Build history of the part. All positions in model axes, mm. A direction names the side the tool comes from. Coordinates: 2 decimals unless noted, no trailing zeros. Loops run counter-clockwise (first coordinate to the right, second up) from the corner with the lowest first, then second, coordinate; pieces in that order, holes last. Notation, with made-up numbers: (86, 56) - (133, 56) arc R18 ccw to (133, 90) - close; hole circle Ø4 at (15, 14). An arc over 180 degrees is marked (long way). One line per item, written item: value.
```python
from build123d import *

# Parameters (mm, degrees)
SKETCH2_R           = 10
BOSS_EXTRUDE1_DEPTH = 8
SKETCH3_R           = 12.5
SKETCH3_R_2         = 7.5
BOSS_EXTRUDE2_DEPTH = 50
BOSS_EXTRUDE3_START = 10
SKETCH4_R           = 12.5
SKETCH4_R_2         = 7.5
BOSS_EXTRUDE3_DEPTH = 10
BOSS_EXTRUDE4_DEPTH = 40
CUT_EXTRUDE1_DEPTH  = 72.52071964
FILLET1_R           = 3


with BuildPart() as part:
    # Sketch2 → Boss-Extrude1 (new body)
    with BuildSketch(Plane(origin=(0, 0, 0), x_dir=(1, 0, 0), z_dir=(0, 1, 0))):
        with BuildLine():
            Line((0, 27.802301255), (0, -12.197698745))
            Line((0, -12.197698745), (19.5, -12.197698745))
            ThreePointArc((19.5, -12.197698745), (39.5, 7.802301255), (19.5, 27.802301255))
            Line((19.5, 27.802301255), (0, 27.802301255))
        make_face()
        with Locations(Location((19.5, 7.802301255, 0), (0, 0, 270))):
            Circle(SKETCH2_R, mode=Mode.SUBTRACT)
    extrude(amount=-BOSS_EXTRUDE1_DEPTH)

    # Sketch3 → Boss-Extrude2 (add)
    with BuildSketch(Plane.XY.offset(12.197698745)):
        with Locations((-8.910855114, -4)):
            Circle(SKETCH3_R)
        with Locations((-8.910855114, -4)):
            Circle(SKETCH3_R_2, mode=Mode.SUBTRACT)
    extrude(amount=-BOSS_EXTRUDE2_DEPTH)

    # Sketch4 → Boss-Extrude3 (add)
    with BuildSketch(Plane.XY.offset(12.197698745).offset(BOSS_EXTRUDE3_START)):
        with Locations((-8.910855114, -4)):
            Circle(SKETCH4_R)
        with Locations((-8.910855114, -4)):
            Circle(SKETCH4_R_2, mode=Mode.SUBTRACT)
    extrude(amount=-BOSS_EXTRUDE3_DEPTH)

    # Sketch6 → Boss-Extrude4 (add)
    with BuildSketch(Plane.XY.offset(12.197698745)):
        Polygon((-18.032516938, -3.352408244), (-55.511163409, 18.285898385), (-51.511163409, 25.214101615), (-14.032516938, 3.575794986), align=None)
    extrude(amount=-BOSS_EXTRUDE4_DEPTH)

    # Sketch7 → Cut-Extrude1 (cut, through all)
    with BuildSketch(Plane(origin=(-1.959764586, -3.394411834, 0), x_dir=(0.866025403784438, -0.500000000000001, 0), z_dir=(0.500000000000001, 0.866025403784438, 0))):
        with BuildLine():
            Line((-47.217026898, 12.802301255), (-27.217026898, 12.802301255))
            ThreePointArc((-27.217026898, 12.802301255), (-22.217026898, 7.802301255), (-27.217026898, 2.802301255))
            Line((-27.217026898, 2.802301255), (-47.217026898, 2.802301255))
            ThreePointArc((-47.217026898, 2.802301255), (-52.217026898, 7.802301255), (-47.217026898, 12.802301255))
        make_face()
    extrude(amount=-CUT_EXTRUDE1_DEPTH, mode=Mode.SUBTRACT)

    # Fillet1
    fillet1_edges = [part.edges().sort_by_distance(p)[0] for p in [
        (-53.511163409, 21.75, -27.802301255),
        (-53.511163409, 21.75, 12.197698745),
    ]]
    fillet(fillet1_edges, radius=FILLET1_R)


solid = part.part
```
Item 1: Pull direction Z, two halves, no side cores. Call faces 1 (the face through (29.415, -3.944, -9.104)), 2 (the face through (25, -8, 1)), 3 (the face through (-52.7, 21.35, 11.34)), 4 (the face through (-49.15, 19.3, -7.69)): released by +Z, released by -Z, zero draft, split by the parting line, or undercut.
Check result:
face 1: undercut
face 2: zero draft
face 3: released by +Z
face 4: undercut
Item 2: Cut at D-D, the plane y = -9. Write the cut outline in (x, z), then the cut area to 3 significant figures.
Check result:
outline: (-20.37, -37.8) - (-14.5, -37.8) - (-14.5, 22.2) - (-20.37, 22.2) - close; (-3.32, -37.8) - (2.55, -37.8) - (2.55, 22.2) - (-3.32, 22.2) - close
area: 704 mm^2
Item 3: Cut at B-B, the plane x = -4. Write the cut outline in (y, z), then the cut area to 3 significant figures.
Check result:
outline: (-15.49, -37.8) - (-9.67, -37.8) - (-9.67, 22.2) - (-15.49, 22.2) - close; (1.67, -37.8) - (7.49, -37.8) - (7.49, 22.2) - (1.67, 22.2) - close
area: 699 mm^2
Item 4: Probe probe 1 along Z at (x, y) = (19, -2); probe 2 along Y at (x, z) = (15, -21); probe 3 along X at (y, z) = (-9.5, -33.5). List the from-to ranges inside material, lowest first. Write a range as from..to.
Check result:
probe 1: z = -27.8..-17.79, 2.19..12.2
probe 2: y = -8..0
probe 3: x = -20.14..-14.01, -3.81..2.31
Item 5: Drop flat-ended pins along their axis: P1, Ø8, axis at y = -3, z = 7, coming from the +X side; P2, Ø18.5, axis at x = -32.5, y = 9, coming from the +Z side; P3, Ø6, axis at x = 20.5, y = 2, coming from the -Z side. Give the stop position or say it passes through.
Check result:
P1: stops at x = 36.33
P2: stops at z = 12.2
P3: stops at z = -27.8
Item 6: Tool access for faces 5 (the face through (-9, -12, 22.198)), 6 (the face through (-34.58, 15.44, -16.41)): list every direction of +Z, -Z, +X, -X, +Y, -Y with a clear straight run to the whole face (end or side of a thin tool).
Check result:
face 5: +Z, +X, -X, +Y, -Y
face 6: +Z, -Z, +Y
Item 7: Cut at C-C, the plane z = -9. Write the cut outline in (x, y), then the cut area to 3 significant figures.
Check result:
outline: (-55.51, 18.29) - (-51.05, 15.71) - (-47.05, 22.64) - (-51.51, 25.21) - close; (-25.33, 0.86) - (-21.17, -1.54) arc R12.5 ccw to (2.93, -8) - (9.57, -8) - (9.57, 0) - (2.93, 0) arc R12.5 ccw to (-17.17, 5.39) - (-21.33, 7.79) - close; (29.43, -8) - (39.46, -8) - (39.46, 0) - (29.43, 0) - close; hole circle Ø15 at (-8.91, -4)
area: 520 mm^2
Item 8: Cut at A-A, the plane y = -4. Write the cut outline in (x, z), then the cut area to 3 significant figures.
Check result:
outline: (-21.41, -37.8) - (-16.41, -37.8) - (-16.41, 22.2) - (-21.41, 22.2) - close; (-1.41, -37.8) - (3.59, -37.8) - (3.59, -27.8) - (19.5, -27.8) arc R20 ccw to (19.5, 12.2) - (3.59, 12.2) - (3.59, 22.2) - (-1.41, 22.2) - close; hole circle Ø20 at (19.5, -7.8)
area: 1,550 mm^2
